from build123d import *

# Parameters (mm, degrees)
SKETCH1_R            = 3.96875
SKETCH1_R_2          = 2
BOSS_EXTRUDE1_DEPTH  = 3.175
M2_CLEARANCE_HOLE1_D = 2.4


with BuildPart() as part:
    # Sketch1 → Boss-Extrude1 (new body)
    with BuildSketch(Plane(origin=(0, 0, 0), x_dir=(1, 0, 0), z_dir=(0, 1, 0))):
        with BuildLine():
            Line((-7.741931284, 6.25), (-40, 6.25))
            ThreePointArc((-40, 6.25), (-46.25, 0), (-40, -6.25))
            Line((-40, -6.25), (-7.741931284, -6.25))
            ThreePointArc((-7.741931284, -6.25), (-5.537138524, -6.496083408), (-3.440858348, -7.222222222))
            ThreePointArc((-3.440858348, -7.222222222), (8, 0), (-3.440858348, 7.222222222))
            ThreePointArc((-3.440858348, 7.222222222), (-5.537138524, 6.496083408), (-7.741931284, 6.25))
        make_face()
        with Locations(Location((-40, 0, 0), (0, 0, 270))):
            Circle(SKETCH1_R, mode=Mode.SUBTRACT)
        with Locations(Location((0, 0, 0), (0, 0, 270))):
            Circle(SKETCH1_R_2, mode=Mode.SUBTRACT)
    extrude(amount=BOSS_EXTRUDE1_DEPTH)

    # M2 Clearance Hole1 (through all)
    with Locations(Plane(origin=(0, 3.175, 0), x_dir=(1, 0, 0), z_dir=(0, 1, 0))):
        with Locations((-4.5, 0), (0, 4.5), (4.5, 0), (0, -4.5)):
            Hole(M2_CLEARANCE_HOLE1_D / 2)


solid = part.part
Input: part model. Units: mm. Frame: model coordinates. A direction names the side the tool comes from. Give positions to 0.01 mm unless a question says otherwise; leave off trailing zeros. Order: outer loops, then holes, each group sorted by start corner. A loop starts at its lowest first (then second) coordinate and runs counter-clockwise, first axis right, second up. Notation, with made-up numbers: M 62,-25.5 L 71,-25.5 A14 cw 71,-9.5 Z; hole C -9,75 d5. An arc over 180 degrees is marked long. Answer as a JSON object with one key per item and string values.
1. Ray query, line 1 (X direction, y = 0.4, z = 1.5); line 2 (Z direction, x = 4, y = 0.15); line 3 (X direction, y = 2.2, z = 4.25). Return the intervals inside material, ascending. Write a range as [from, to].
Result sheet:
{"line 1": "[-46.07, -43.67], [-36.33, -1.32], [1.32, 7.86]", "line 2": "[-6.93, -1.09], [1.09, 6.93]", "line 3": "[-44.58, -1.17], [1.17, 6.78]"}
2. First-contact query: P1, Ø1.5, axis at y = 0.5, z = 3.5, coming from the -X side; P2, Ø1, axis at x = -19.5, y = 1, coming from the -Z side; P3, Ø1.9, axis at x = -4.5, z = 0, coming from the -Y side. Flat tips, straight axial feed; report the tip coordinate or a pass-through.
Result sheet:
{"P1": "x = -45.61", "P2": "z = -6.25", "P3": "through"}
3. Cut plane C-C, the plane y = 2.3. Output: boundary loops of the cut face in (x, z), and give its area (3 significant figures).
Result sheet:
{"outline": "M -40,-6.25 L -7.74,-6.25 A10 cw -3.44,-7.22 A8 ccw long -3.44,7.22 A10 cw -7.74,6.25 L -40,6.25 A6.25 ccw Z; hole C -40,0 d7.94; hole C -4.5,0 d2.4; hole C 0,0 d4; hole C 0,-4.5 d2.4; hole C 0,4.5 d2.4; hole C 4.5,0 d2.4", "area": "595 mm²"}
4. Cut plane B-B, the plane z = 0. Output: boundary loops of the cut face in (x, y) (3 decimals), and give its area (3 significant figures).
Result sheet:
{"outline": "M -46.25,0 L -43.969,0 L -43.969,3.175 L -46.25,3.175 Z; M -36.031,0 L -5.7,0 L -5.7,3.175 L -36.031,3.175 Z; M -3.3,0 L -2,0 L -2,3.175 L -3.3,3.175 Z; M 2,0 L 3.3,0 L 3.3,3.175 L 2,3.175 Z; M 5.7,0 L 8,0 L 8,3.175 L 5.7,3.175 Z", "area": "119 mm²"}
5. Cut plane D-D, the plane z = -4.5. Output: boundary loops of the cut face in (x, y) (3 decimals), and give its area (3 significant figures).
Result sheet:
{"outline": "M -44.337,0 L -1.2,0 L -1.2,3.175 L -44.337,3.175 Z; M 1.2,0 L 6.614,0 L 6.614,3.175 L 1.2,3.175 Z", "area": "154 mm²"}
6. Reachability of faces 4 (the flat face through (-24, 2, -6.25)), 5 (the flat face through (-20, 0, 0)) from +Z, -Z, +X, -X, +Y, -Y: full face, straight path, thin tool, end or side. Return the list, or none.
Result sheet:
{"face 4": "-Z, -X, +Y, -Y", "face 5": "+Z, -Z, +X, -X, -Y"}
7. Cut plane A-A, the plane x = 0. Output: boundary loops of the cut face in (y, z) (3 decimals), and give its area (3 significant figures).
Result sheet:
{"outline": "M 0,-8 L 3.175,-8 L 3.175,-5.7 L 0,-5.7 Z; M 0,-3.3 L 3.175,-3.3 L 3.175,-2 L 0,-2 Z; M 0,2 L 3.175,2 L 3.175,3.3 L 0,3.3 Z; M 0,5.7 L 3.175,5.7 L 3.175,8 L 0,8 Z", "area": "22.9 mm²"}
8. Pull-direction query (Z, two-part tool) for faces 1 (the flat face through (-24, 2, 6.25)), 2 (the cylindrical face through (-5.507, 1.565, -6.503)), 3 (the cylindrical face through (5.7, 1.57, -0.05)); classes: +Z half, -Z half, draft (parallel to the pull), parting line (faces both ways), or undercut.
Result sheet:
{"face 1": "+Z half", "face 2": "-Z half", "face 3": "undercut"}
